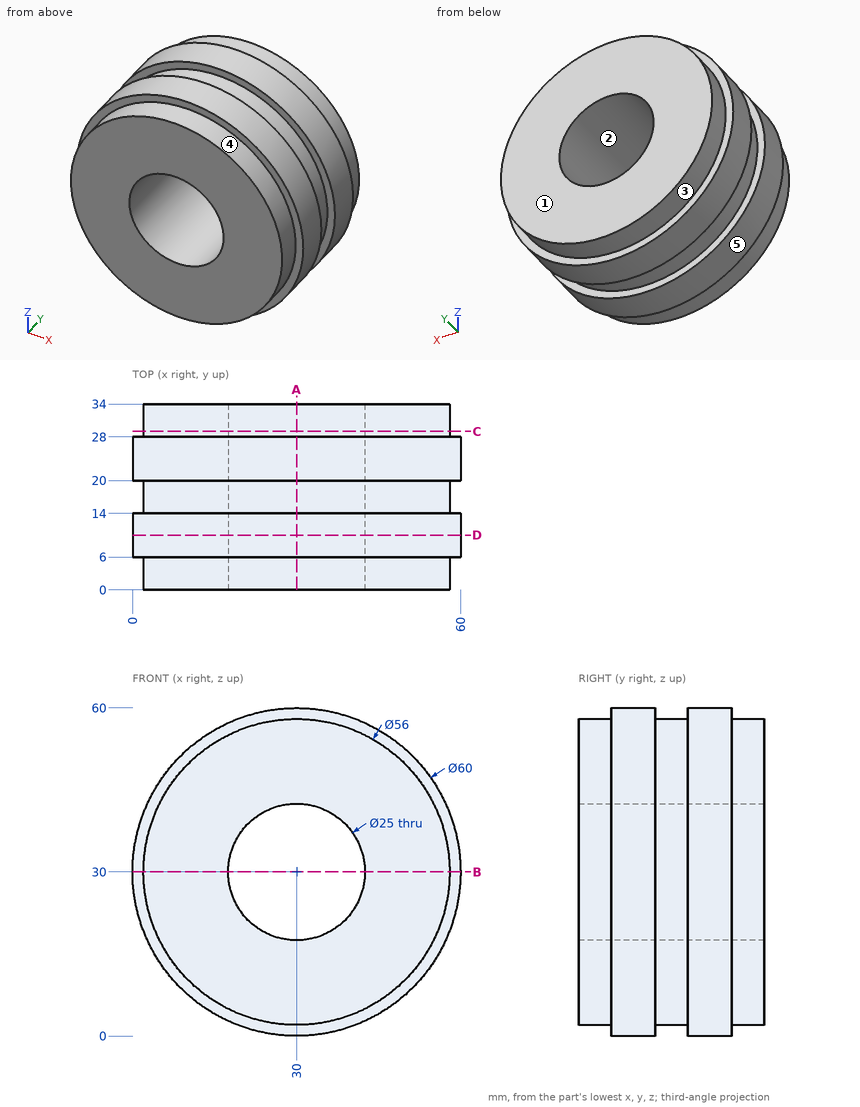
Input: dimensioned drawing with shaded views. Units: mm. Origin: part minimum x, y, z. A direction names the side the tool comes from. Round coordinates to 2 decimals unless told otherwise and drop trailing zeros. Loops run counter-clockwise (first coordinate to the right, second up) from the corner with the lowest first, then second, coordinate; pieces in that order, holes last. Notation, with made-up numbers: (3, -26) -> (47, -26) arc R27 cw to (47, 6) -> close; hole circle Ø5 at (80, 18). An arc over 180 degrees is marked (long way). Use one line per item in the form item = value. Start each with the question number.
1) Line query: L1, parallel to X at y = 21, z = 30; L2, parallel to X at y = 19, z = 30; L3, parallel to Y at x = 55.5, z = 42. Output: solid intervals per line, ascending.
2) Draft query along Z for the marked faces 1, 2 and 3. Return one class per face: released by +Z, released by -Z, zero draft, split by the parting line, or undercut.
3) Section A-A on x = 30. Output: boundary loops of the cut face in (y, z).
4) Section C-C on y = 29. Output: boundary loops of the cut face in (x, z).
5) Section B-B on z = 30. Output: boundary loops of the cut face in (x, y), then the cut area to 3 significant figures.
6) Access query for the marked faces 4 and 5. Directions: +Z, -Z, +X, -X, +Y, -Y. A direction counts if a zero-diameter tool reaches every point of the face in a straight line with its end or side. Return the directions, or none.
7) Section D-D on y = 10. Output: boundary loops of the cut face in (x, z), then the cut area to 3 significant figures.
8) First-contact query: P1, Ø8, axis at x = 45.5, y = 5.5, coming from the +Z side; P2, Ø5, axis at y = 6.5, z = 48, coming from the +X side; P3, Ø5, axis at x = 34.5, y = 14, coming from the +Z side. Flat tips, straight axial feed; report the tip coordinate or a pass-through.
Response:
q1.L1 = 0 to 17.5, 42.5 to 60
q1.L2 = 2 to 17.5, 42.5 to 58
q1.L3 = 6 to 14, 20 to 28
q2.face_1 = zero draft
q2.face_2 = undercut
q2.face_3 = split by the parting line
q3.outline = (0, 2) -> (6, 2) -> (6, 0) -> (14, 0) -> (14, 2) -> (20, 2) -> (20, 0) -> (28, 0) -> (28, 2) -> (34, 2) -> (34, 17.5) -> (0, 17.5) -> close; (0, 42.5) -> (34, 42.5) -> (34, 58) -> (28, 58) -> (28, 60) -> (20, 60) -> (20, 58) -> (14, 58) -> (14, 60) -> (6, 60) -> (6, 58) -> (0, 58) -> close
q4.outline = circle Ø56 at (30, 30); hole circle Ø25 at (30, 30)
q5.outline = (0, 6) -> (2, 6) -> (2, 0) -> (17.5, 0) -> (17.5, 34) -> (2, 34) -> (2, 28) -> (0, 28) -> (0, 20) -> (2, 20) -> (2, 14) -> (0, 14) -> close; (42.5, 0) -> (58, 0) -> (58, 6) -> (60, 6) -> (60, 14) -> (58, 14) -> (58, 20) -> (60, 20) -> (60, 28) -> (58, 28) -> (58, 34) -> (42.5, 34) -> close
q5.area = 1,120 mm^2
q6.face_4 = -Y
q6.face_5 = +Y, -Y
q7.outline = circle Ø60 at (30, 30); hole circle Ø25 at (30, 30)
q7.area = 2,340 mm^2
q8.P1 = 57.7
q8.P2 = 55.69
q8.P3 = 59.93
